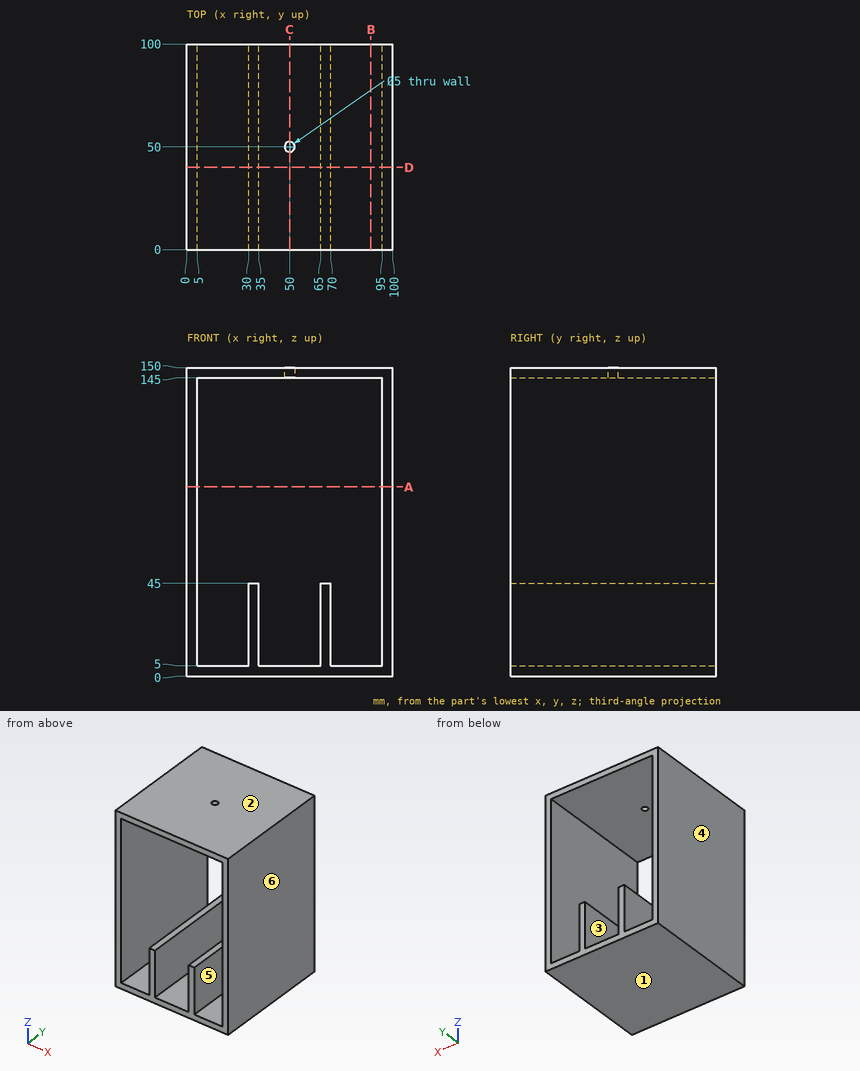
Drawing for the job (mm, zero at the part's lowest x, y, z). A direction names the side the tool comes from. Give positions to 0.01 mm unless a question says otherwise; leave off trailing zeros. Order: outer loops, then holes, each group sorted by start corner. A loop starts at its lowest first (then second) coordinate and runs counter-clockwise, first axis right, second up. Notation, with made-up numbers: M -24.5,50.25 L 5.5,50.25 A20 cw 5.5,87.25 Z; hole C -19,-8 d9. An arc over 180 degrees is marked long. Use a Markdown table: item, result. Add a question column.
(1) Saw through at B-B, the plane x = 89.5. Give the cut face in (y, z).
(2) Mould opens along Z. For the marked faces 1, 2, 3 and 4 say: +Z half, -Z half, draft (parallel to the pull), parting line (faces both ways), or undercut.
(3) Saw through at A-A, the plane z = 92. Give the cut face in (x, y), and give its area (3 significant figures).
(4) Saw through at D-D, the plane y = 40. Give the cut face in (x, z), and give its area (3 significant figures).
(5) 3-axis set-ups, long thin cutter, end or side, ignore diameter. For the marked faces 5 and 6: which of +Z, -Z, +X, -X, +Y, -Y reach the whole face in a straight line?
(6) Drop a flat-ended pin along its axis: P1, Ø4.5, axis at x = 50, y = 50, coming from the +Z side. Give the stop position or say it passes through.
(7) Probe line 1 along X through (y, z) = (62, 7.5); line 2 along X through (y, z) = (24, 135); line 3 along Z through (x, y) = (15, 35). List the from-to ranges inside material, lowest first. Write a range as [from, to].
(8) Saw through at C-C, the plane x = 50. Give the cut face in (y, z), and give its area (3 significant figures).
Answer key:
| question | item | result |
|---|---|---|
| 1 | outline | M 0,0 L 100,0 L 100,5 L 0,5 Z; M 0,145 L 100,145 L 100,150 L 0,150 Z |
| 2 | face 1 | -Z half |
| 2 | face 2 | +Z half |
| 2 | face 3 | undercut |
| 2 | face 4 | draft |
| 3 | outline | M 0,0 L 5,0 L 5,100 L 0,100 Z; M 95,0 L 100,0 L 100,100 L 95,100 Z |
| 3 | area | 1,000 mm^2 |
| 4 | outline | M 0,0 L 100,0 L 100,150 L 0,150 Z; hole M 5,5 L 30,5 L 30,45 L 35,45 L 35,5 L 65,5 L 65,45 L 70,45 L 70,5 L 95,5 L 95,145 L 5,145 Z |
| 4 | area | 2,800 mm^2 |
| 5 | face 5 | +Y, -Y |
| 5 | face 6 | +Z, -Z, +X, +Y, -Y |
| 6 | P1 | z = 5 |
| 7 | line 1 | [0, 5], [30, 35], [65, 70], [95, 100] |
| 7 | line 2 | [0, 5], [95, 100] |
| 7 | line 3 | [0, 5], [145, 150] |
| 8 | outline | M 0,0 L 100,0 L 100,5 L 0,5 Z; M 0,145 L 47.5,145 L 47.5,150 L 0,150 Z; M 52.5,145 L 100,145 L 100,150 L 52.5,150 Z |
| 8 | area | 975 mm^2 |
